from build123d import *

# Parameters (mm, degrees)
SKETCH1_W           = 150
SKETCH1_H           = 20
BOSS_EXTRUDE1_DEPTH = 10
SKETCH2_R           = 3
CUT_EXTRUDE1_DEPTH  = 10
SKETCH3_W           = 23
SKETCH3_H           = 25
BOSS_EXTRUDE2_DEPTH = 10
SKETCH4_R           = 2.5
CUT_EXTRUDE2_DEPTH  = 480.576193501
SKETCH5_W           = 10
SKETCH5_H           = 35
BOSS_EXTRUDE3_DEPTH = 50


with BuildPart() as part:
    # Sketch1 → Boss-Extrude1 (new body)
    with BuildSketch(Plane(origin=(0, 0, 0), x_dir=(1, 0, 0), z_dir=(0, 1, 0))):
        with Locations((-2472.770700637, 441.167728238)):
            Rectangle(SKETCH1_W, SKETCH1_H)
    extrude(amount=BOSS_EXTRUDE1_DEPTH)

    # Sketch2 → Cut-Extrude1 (cut)
    with BuildSketch(Plane(origin=(0, 10, 0), x_dir=(1, 0, 0), z_dir=(0, 1, 0))):
        with Locations(Location((-2407.770700637, 441.167728238, 0), (0, 0, 270))):
            Circle(SKETCH2_R)
    extrude(amount=-CUT_EXTRUDE1_DEPTH, mode=Mode.SUBTRACT)

    # Sketch3 → Boss-Extrude2 (add)
    with BuildSketch(Plane.ZY.offset(2547.770700637)):
        with Locations((-442.667728238, 22.5)):
            Rectangle(SKETCH3_W, SKETCH3_H)
    extrude(amount=-BOSS_EXTRUDE2_DEPTH)

    # Sketch4 → Cut-Extrude2 (cut, through all)
    with BuildSketch(Plane.ZY.offset(2547.770700637)):
        with Locations((-448.417728238, 25)):
            Circle(SKETCH4_R)
        with Locations((-438.417728238, 25)):
            Circle(SKETCH4_R)
    extrude(amount=-CUT_EXTRUDE2_DEPTH, mode=Mode.SUBTRACT)

    # Sketch5 → Boss-Extrude3 (add)
    with BuildSketch(Plane.XY.offset(-431.167728238)):
        with Locations((-2542.770700637, 17.5)):
            Rectangle(SKETCH5_W, SKETCH5_H)
    extrude(amount=BOSS_EXTRUDE3_DEPTH)


solid = part.part
For this review, take the finished solid that the model builds, in its own axes (mm). A direction names the side the tool comes from. Round coordinates to 2 decimals unless told otherwise and drop trailing zeros. Loops run counter-clockwise (first coordinate to the right, second up) from the corner with the lowest first, then second, coordinate; pieces in that order, holes last. Notation, with made-up numbers: (37.25, 86) - (96.25, 86) arc R17 cw to (96.25, 109) - close; hole circle Ø1 at (7.25, 32.5). An arc over 180 degrees is marked (long way). One line per question, with ' | ' between items.
Q1. Tool access review of faces 1 (the flat face through (-2469, 10, -441)), 2 (the flat face through (-2469, 5, -431.168)), 3 (the cylindrical face through (-2542.841, 25.11, -450.915)): name each direction out of +Z, -Z, +X, -X, +Y, -Y from which nothing blocks a thin tool from reaching the whole face with its end or side.
Taken from the geometry:
face 1: +Z, -Z, +X, +Y | face 2: +Z, +X, +Y, -Y | face 3: +X, -X
Q2. Take a section at C-C (y = 19). Give the boundary of the cut face in (x, z), and give its area (3 significant figures).
Taken from the geometry:
outline: (-2547.77, -454.17) - (-2537.77, -454.17) - (-2537.77, -381.17) - (-2547.77, -381.17) - close | area: 730 mm²
Q3. Take a section at D-D (z = -394). Give the boundary of the cut face in (x, y), and give its area (3 significant figures).
Taken from the geometry:
outline: (-2547.77, 0) - (-2537.77, 0) - (-2537.77, 35) - (-2547.77, 35) - close | area: 350 mm²
Q4. Take a section at A-A (y = 25). Give the boundary of the cut face in (x, z).
Taken from the geometry:
outline: (-2547.77, -454.17) - (-2537.77, -454.17) - (-2537.77, -450.92) - (-2547.77, -450.92) - close; (-2547.77, -445.92) - (-2537.77, -445.92) - (-2537.77, -440.92) - (-2547.77, -440.92) - close; (-2547.77, -435.92) - (-2537.77, -435.92) - (-2537.77, -381.17) - (-2547.77, -381.17) - close
Q5. Take a section at B-B (z = -447.5). Give the boundary of the cut face in (x, y), and give its area (3 significant figures).
Taken from the geometry:
outline: (-2547.77, 0) - (-2397.77, 0) - (-2397.77, 10) - (-2537.77, 10) - (-2537.77, 22.67) - (-2547.77, 22.67) - close; (-2547.77, 27.33) - (-2537.77, 27.33) - (-2537.77, 35) - (-2547.77, 35) - close | area: 1,700 mm²
Q6. For line 1 along Z through (x, y) = (-2407.5, 5); line 2 along X through (y, z) = (28.5, -448); line 3 along Y through (x, z) = (-2439, -446), list the stretches that pass through material, from the lowest coordinate up. Write a range as [from, to].
Taken from the geometry:
line 1: z = [-451.17, -444.16], [-438.18, -431.17] | line 2: x = [-2547.77, -2537.77] | line 3: y = [0, 10]
Q7. The part is to be moulded in two halves that separate along Y. For faces 4 (the cylindrical face through (-2542.841, 25.11, -440.915)), 5 (the flat face through (-2543, 10, -453)), 6 (the flat face through (-2397.771, 5, -441)), say which applies: released by +Y, released by -Y, zero draft, split by the parting line, or undercut.
Taken from the geometry:
face 4: undercut | face 5: released by -Y | face 6: zero draft
Q8. For pin 1 (11 mm diameter, centred on x = -2476.5, y = 5, fed in from -Z); pin 2 (1.5 mm diameter, centred on x = -2543.5, z = -452, fed in from -Y); pin 3 (22 mm diameter, centred on x = -2494, z = -439.5, fed in from +Y), all flat-tipped, find the tip position at first contact; note any pin that passes through.
Taken from the geometry:
pin 1: stops at z = -451.17 | pin 2: stops at y = 10 | pin 3: stops at y = 10
